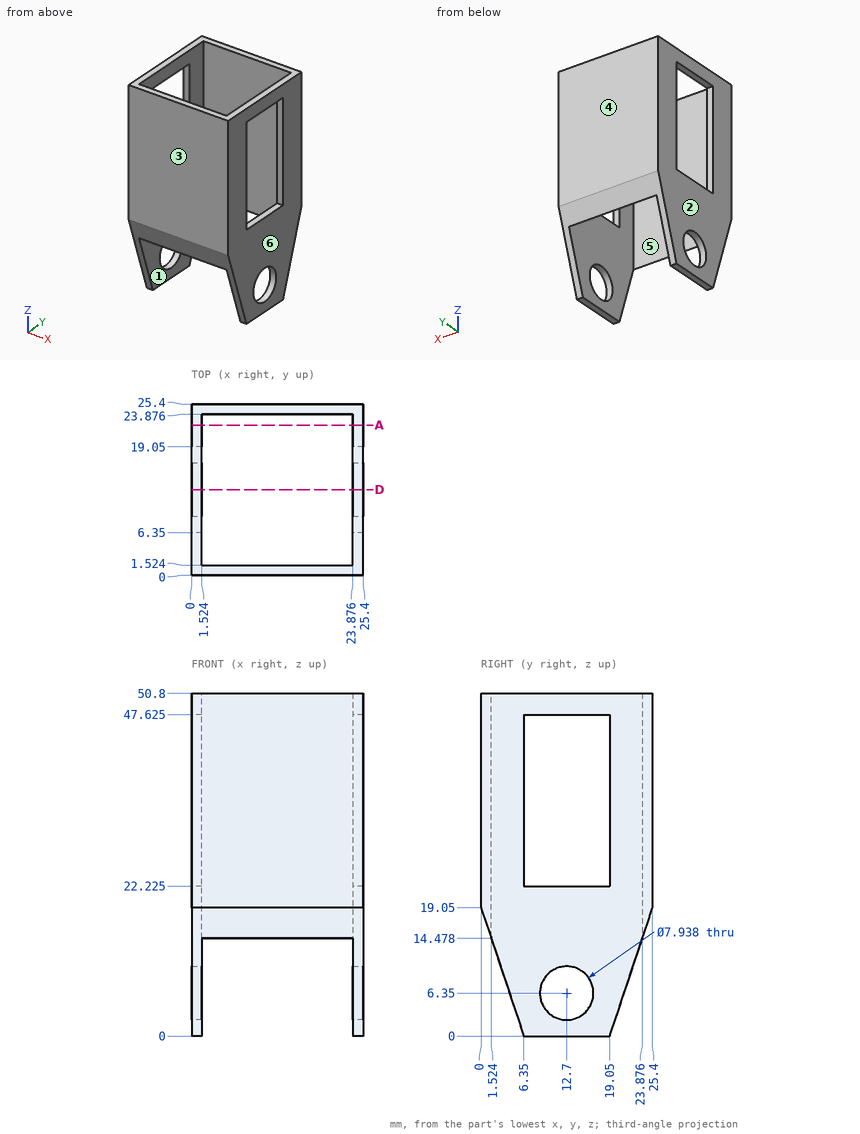
Study the drawing (mm; zero at the part's minimum x, y, z) and answer. A direction names the side the tool comes from. Give positions to 0.01 mm unless a question says otherwise; leave off trailing zeros. Write each loop counter-clockwise with the first axis right and the second up, starting at its lowest first coordinate (ties: lowest second). Pieces come first, ordered by that corner, then holes. Notation, with made-up numbers: (44.5, 79) - (76.5, 79) arc R33 cw to (76.5, 114) - close; hole circle Ø5 at (29, 67). An arc over 180 degrees is marked (long way). One line per question, with ' | ' between items. Start each with the question number.
1. Straight lines are drawn through the part: line 1 (X direction, y = 7.5, z = 14) (1 decimal); line 2 (Z direction, x = 1, y = 9.75) (1 decimal). For each, find the intervals that lie inside material, in ascending order.
2. Section A-A, the plane y = 22.25 is taken. Determine the outline of the cut face in (x, z) (1 decimal).
3. Determine the mould class of the marked faces 1, 2, 3 and 4 for opening direction Y: +Y half, -Y half, draft (parallel to the pull), parting line (faces both ways), or undercut.
4. Section D-D, the plane y = 12.7 is taken. Determine the outline of the cut face in (x, z) (1 decimal).
5. For the marked faces 5 and 6, determine the directions among +Z, -Z, +X, -X, +Y, -Y from which every point of the face is accessible in a straight line to the end or side of a thin tool.
Result:
1) line 1: x = 0 to 1.5, 23.9 to 25.4 | line 2: z = 0 to 3.7, 9 to 22.2, 47.6 to 50.8
2) outline: (0, 9.6) - (1.5, 9.6) - (1.5, 50.8) - (0, 50.8) - close; (23.9, 9.6) - (25.4, 9.6) - (25.4, 50.8) - (23.9, 50.8) - close
3) face 1: undercut | face 2: draft | face 3: -Y half | face 4: +Y half
4) outline: (0, 0) - (1.5, 0) - (1.5, 2.4) - (0, 2.4) - close; (0, 10.3) - (1.5, 10.3) - (1.5, 22.2) - (0, 22.2) - close; (0, 47.6) - (1.5, 47.6) - (1.5, 50.8) - (0, 50.8) - close; (23.9, 0) - (25.4, 0) - (25.4, 2.4) - (23.9, 2.4) - close; (23.9, 10.3) - (25.4, 10.3) - (25.4, 22.2) - (23.9, 22.2) - close; (23.9, 47.6) - (25.4, 47.6) - (25.4, 50.8) - (23.9, 50.8) - close
5) face 5: +Z, -Z | face 6: +Z, -Z, +X, +Y, -Y
